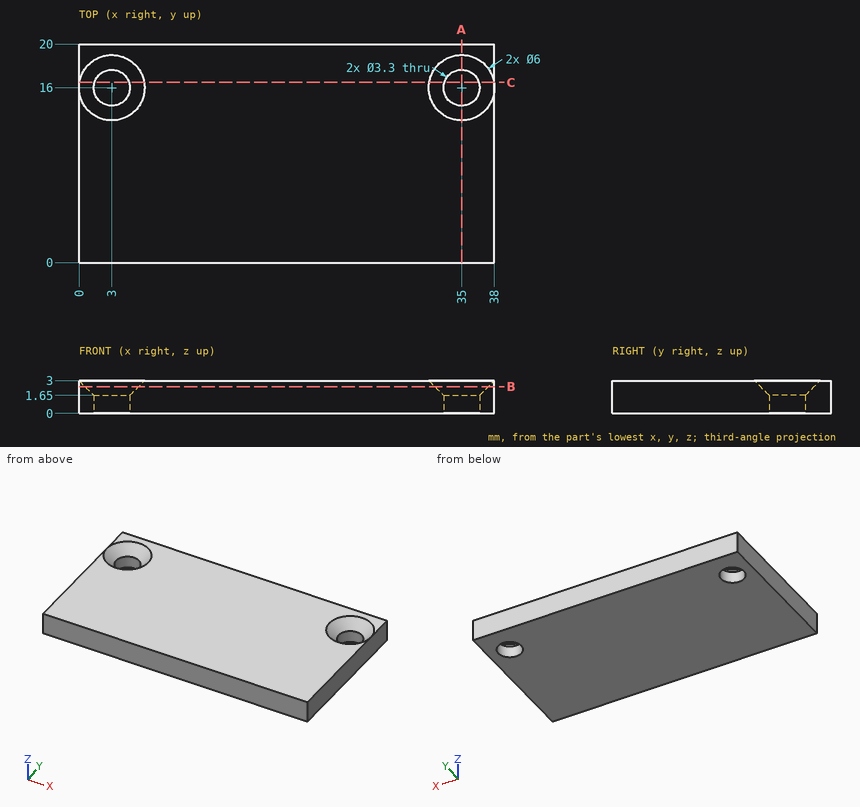
Study the drawing (mm; zero at the part's minimum x, y, z) and answer. Give positions to 0.01 mm unless a question says otherwise; leave off trailing zeros. Loops run counter-clockwise (first coordinate to the right, second up) from the corner with the lowest first, then second, coordinate; pieces in that order, holes last. Notation, with made-up numbers: (52.5, 26.25) - (102.5, 26.25) arc R17 cw to (102.5, 48.25) - close; hole circle Ø2 at (84, 52). An arc over 180 degrees is marked (long way). Use CSV: the item, a comma, the result in double quotes. Start each with the question number.
(1) Find section C-C, the plane y = 16.5. Count the separate pieces of the cut face and the enclosed holes in it, plus the area to 3 significant figures.
(2) Find section A-A, the plane x = 35. Determine the outline of the cut face in (y, z), plus the area to 3 significant figures.
(3) Find section B-B, the plane z = 2.45. Determine the outline of the cut face in (x, y).
(4) This flat-tipped pin is pushed along its axis until it touches: pin 1 (5.5 mm diameter, centred on x = 35, y = 16, fed in from -Z). Where does it stop, or does it pass through?
(5) Find the intervals of material crossed by L1, parallel to X at y = 16, z = 1; L2, parallel to Y at x = 35, z = 0.7; L3, parallel to Y at x = 33.5, z = 2.4, in increasing order.
Results found:
1,separate pieces,"3"
1,enclosed holes,"0"
1,area,"91.4 mm^2"
2,outline,"(0, 0) - (14.35, 0) - (14.35, 1.65) - (13, 3) - (0, 3) - close; (17.65, 0) - (20, 0) - (20, 3) - (19, 3) - (17.65, 1.65) - close"
2,area,"48.3 mm^2"
3,outline,"(0, 0) - (38, 0) - (38, 20) - (0, 20) - close; hole circle Ø4.9 at (3, 16); hole circle Ø4.9 at (35, 16)"
4,pin 1,"z = 0"
5,L1,"0 to 1.35, 4.65 to 33.35, 36.65 to 38"
5,L2,"0 to 14.35, 17.65 to 20"
5,L3,"0 to 14.13, 17.87 to 20"
